Autodesk Inventor part; units mm, degrees
ref_plane "YZ Plane" through (0, 0, 0) normal (1, 0, 0) x (0, 1, 0)
ref_plane "XZ Plane" through (0, 0, 0) normal (0, 1, 0) x (-1, 0, 0)
ref_plane "XY Plane" through (0, 0, 0) normal (0, 0, 1) x (1, 0, 0)
sketch "Sketch1" plane through (0, 0, 0) normal (0, 0, 1) x (1, 0, 0)
  line L0 (0, 0) -> (-63.5, 0)
  line L1 (-63.5, 0) -> (-63.5, 63.5)
  line L2 (-63.5, 63.5) -> (0, 63.5)
  circle A0 centre (-58.7502, 31.75) radius 2.54
  circle A1 centre (-31.75, 58.7502) radius 2.54
  circle A2 centre (-4.7498, 31.75) radius 2.54
  circle A3 centre (-31.75, 4.7498) radius 2.54
  line L3 (36.9316, 63.5) -> (36.9316, 0)
  line L4 (13.1168, 0) -> (0, 0)
  circle A4 centre (-31.75, 31.75) radius 14.2875
  line L5 (24.2316, 63.5) -> (24.2316, 44.45)
  line L6 (24.2316, 44.45) -> (24.2316, 19.05)
  circle A5 centre (24.2316, 44.45) radius 3.3782
  circle A6 centre (24.2316, 19.05) radius 3.3782
  line L7 (20.8534, 44.45) -> (20.8534, 19.05)
  line L8 (27.6098, 19.05) -> (27.6098, 44.45)
  line L9 (11.5316, 63.5) -> (11.5316, 114.3)
  line L10 (13.1168, 0) -> (13.1168, -25.4)
  line L11 (13.1168, -25.4) -> (36.9316, -25.4)
  line L12 (36.9316, -25.4) -> (36.9316, 0)
  line L13 (11.5316, 114.3) -> (36.9316, 114.3)
  line L14 (36.9316, 114.3) -> (36.9316, 63.5)
  line L15 (0, 63.5) -> (11.5316, 63.5)
  dimension "d0" = 63.5
  dimension "d1" = 63.5
  dimension "d6" = 5.08
  dimension "d7" = 5.08
  dimension "d8" = 5.08
  dimension "d9" = 5.08
  dimension "d11" = 36.9316
  dimension "d12" = 28.575
  dimension "d13" = 12.7
  dimension "d15" = 25.4
  dimension "d16" = 6.7564
  dimension "d17" = 6.7564
  dimension "d23" = 50.8
  dimension "d24" = 25.4
extrude "Plate2" add sketch "Sketch1" along normal blind 3.048 contours L0 L1 L2 L15 L9 L13 L14 L3 L12 L11 L10 L4 | L8 A6 L6 A5 | A5 L6 A6 L7
sketch "Sketch4" plane through (0, 0, 3.048) normal (0, 0, 1) x (1, 0, 0)
  circle A0 centre (24.2316, 19.05) radius 3.3782
  circle A1 centre (24.2316, 44.45) radius 3.3782
  line L0 (-63.5, 63.5) -> (11.5316, 63.5)
  line L1 (24.2316, 44.45) -> (24.2316, 101.6)
  circle A2 centre (24.2316, 101.6) radius 3.3782
  circle A3 centre (24.2316, 73.025) radius 3.3782
  line L2 (24.2316, 19.05) -> (24.2316, -14.605)
  circle A4 centre (24.2316, -14.605) radius 3.3782
  point P0 (0, 0)
  point P1 (20.8534, 44.45)
  point P2 (20.8534, 19.05)
  point P3 (27.6098, 19.05)
  point P4 (27.6098, 44.45)
  dimension "d25" = 57.15
  dimension "d26" = 6.7564
  dimension "d27" = 6.7564
  dimension "d28" = 33.655
  dimension "d29" = 6.7564
extrude "Cut1" cut sketch "Sketch4" against normal blind 3.048
fillet "Corner Round1" radius 19.05 2 edges at (11.5316, 63.5, 1.524) (13.1168, 0, 1.524)
fillet "Corner Round2" radius 6.35 6 edges at (-63.5, 63.5, 1.524) (-63.5, 0, 1.524) (13.1168, -25.4, 1.524) (36.9316, -25.4, 1.524) (36.9316, 114.3, 1.524) (11.5316, 114.3, 1.524)
equation "\"d19\" = Thickness"
equation "\"BendRadius\" = Thickness"
equation "\"BendReliefWidth\" = Thickness"
equation "\"BendReliefDepth\" = 0.5 * Thickness"
equation "\"CornerReliefSize\" = 4 * Thickness"
equation "\"MinimumRemnant\" = 2 * Thickness"
equation "\"TransitionRadius\" = BendRadius"
equation "\"JacobiRadiusSize\" = BendRadius"
equation "\"GapSize\" = Thickness"
equation "\"d10\" = BendRadius"
equation "\"d18\" = BendRadius"
properties part number "M - p80 mount plate" material "Aluminum 6061"
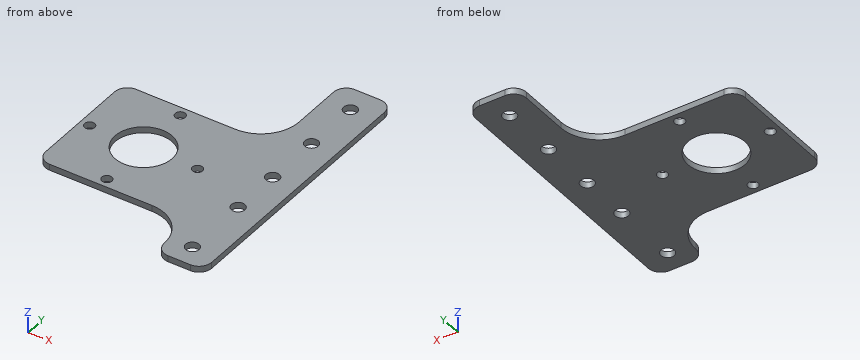
Can you work these out from the model? Positions are in its coordinate system, mm. Give positions to 0.01 mm unless a question says otherwise; leave off trailing zeros. Write each loop counter-clockwise with the first axis right and the second up, starting at its lowest first coordinate (ties: lowest second). Pieces come first, ordered by that corner, then holes. Notation, with made-up numbers: M 58,61.5 L 96,61.5 A27 cw 96,91.5 Z; hole C 89.25,-16.75 d3. An arc over 180 degrees is marked long. Answer in a Markdown table with one row per item. Add a question column.
Item 1: Imagine slicing it at D-D, the plane z = 1.5. State how many separate pieces and enclosed holes the cut face has, plus the area to 3 significant figures.
Item 2: Imagine slicing it at A-A, the plane y = 101.6. Write out the boundary of the cut face in (x, z).
Item 3: Please list where these lines run through material, in increasing order: L1, parallel to Y at x = -32, z = 1.1; L2, parallel to Y at x = -34, z = 1.25; L3, parallel to X at y = 22, z = 0.2.
Item 4: Imagine slicing it at C-C, the plane x = -37.5. Write out the boundary of the cut face in (y, z), plus the area to 3 significant figures.
Item 5: For pin 1 Ø1.5 at (y, z) = (95.5, 1.5) entering from -X; pin 2 Ø4.5 at (x, y) = (-31.75, 4.75) entering from +Z; pin 3 Ø0.9 at (x, z) = (-29, 1) entering from +Y, each with a flat end and sliding along its axis, tell me the tip position at first contact or that it passes through.
Item 6: Imagine slicing it at B-B, the plane y = 31.75. Write out the boundary of the cut face in (x, z), plus the area to 3 significant figures.
Evaluation:
| question | item | result |
|---|---|---|
| 1 | separate pieces | 1 |
| 1 | enclosed holes | 10 |
| 1 | area | 7,470 mm² |
| 2 | outline | M 11.53,0 L 20.85,0 L 20.85,3.05 L 11.53,3.05 Z; M 27.61,0 L 36.93,0 L 36.93,3.05 L 27.61,3.05 Z |
| 3 | L1 | y = 0 to 2.22, 7.28 to 17.46, 46.04 to 56.22, 61.28 to 63.5 |
| 3 | L2 | y = 0 to 3.57, 5.93 to 17.64, 45.86 to 57.57, 59.93 to 63.5 |
| 3 | L3 | x = -63.5 to -42.19, -21.31 to 22.59, 25.88 to 36.93 |
| 4 | outline | M 0,0 L 18.67,0 L 18.67,3.05 L 0,3.05 Z; M 44.83,0 L 63.5,0 L 63.5,3.05 L 44.83,3.05 Z |
| 4 | area | 114 mm² |
| 5 | pin 1 | stops at x = 11.53 |
| 5 | pin 2 | passes through |
| 5 | pin 3 | stops at y = 63.5 |
| 6 | outline | M -63.5,0 L -61.29,0 L -61.29,3.05 L -63.5,3.05 Z; M -56.21,0 L -46.04,0 L -46.04,3.05 L -56.21,3.05 Z; M -17.46,0 L -7.29,0 L -7.29,3.05 L -17.46,3.05 Z; M -2.21,0 L 36.93,0 L 36.93,3.05 L -2.21,3.05 Z |
| 6 | area | 188 mm² |
